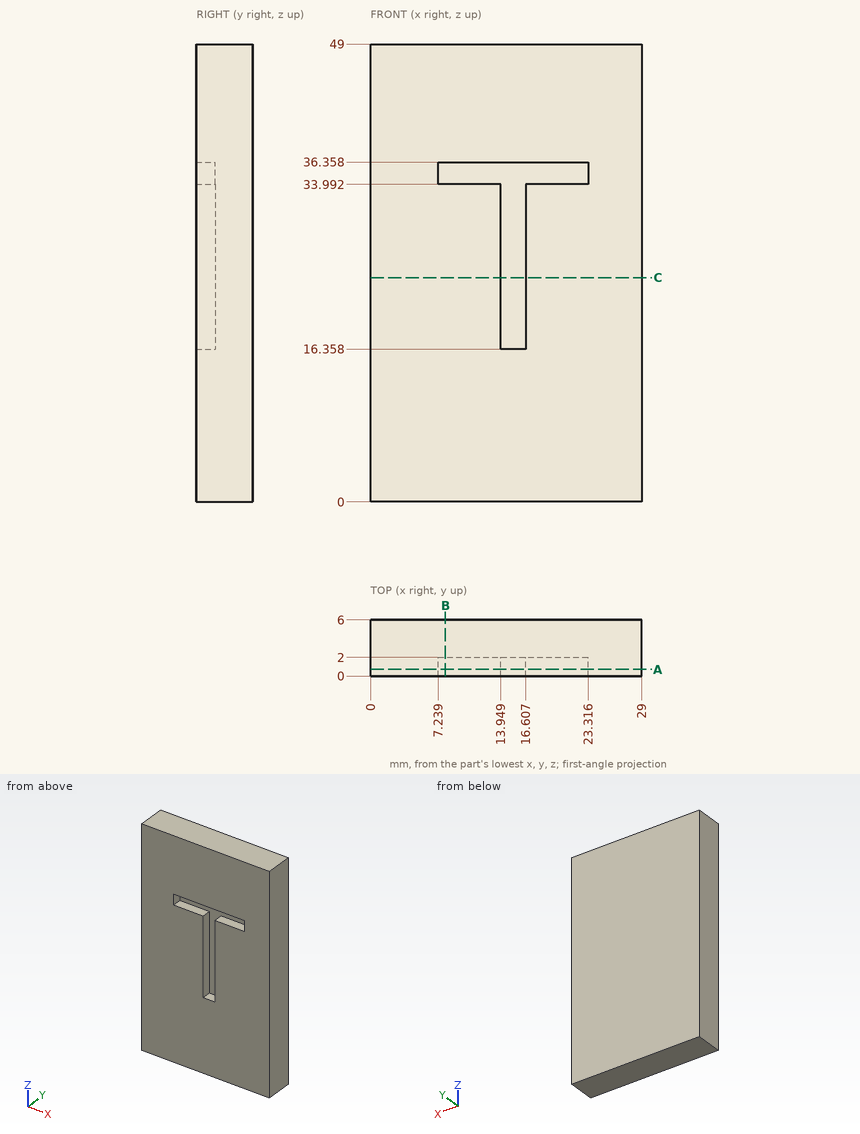
Print and shaded views of the part. All mm, measured from the part's lowest x, y and z. Coordinates: 2 decimals unless noted, no trailing zeros. Order: outer loops, then holes, each group sorted by start corner. A loop starts at its lowest first (then second) coordinate and runs counter-clockwise, first axis right, second up. Notation, with made-up numbers: (-13, 20.5) - (-8, 20.5) arc R20 cw to (-8, 52.5) - close; hole circle Ø5 at (-7, -2). An arc over 180 degrees is marked (long way). Put each result on its own line as item: value.
1. Saw through at B-B (x = 8). Write the cut outline in (y, z), and give its area (3 significant figures).
Answer sheet:
outline: (0, 0) - (6, 0) - (6, 49) - (0, 49) - (0, 36.36) - (2, 36.36) - (2, 33.99) - (0, 33.99) - close
area: 289 mm^2
2. Saw through at C-C (z = 24). Write the cut outline in (x, y), and give its area (3 significant figures).
Answer sheet:
outline: (0, 0) - (13.95, 0) - (13.95, 2) - (16.61, 2) - (16.61, 0) - (29, 0) - (29, 6) - (0, 6) - close
area: 169 mm^2
3. Saw through at A-A (y = 0.7). Write the cut outline in (x, z), and give its area (3 significant figures).
Answer sheet:
outline: (0, 0) - (29, 0) - (29, 49) - (0, 49) - close; hole (7.24, 33.99) - (13.95, 33.99) - (13.95, 16.36) - (16.61, 16.36) - (16.61, 33.99) - (23.32, 33.99) - (23.32, 36.36) - (7.24, 36.36) - close
area: 1,340 mm^2
4. Probe line 1 along X through (y, z) = (1.95, 17); line 2 along Z through (x, y) = (20.5, 1). List the from-to ranges inside material, lowest first. Write a range as [from, to].
Answer sheet:
line 1: x = [0, 13.95], [16.61, 29]
line 2: z = [0, 33.99], [36.36, 49]
